The model under review builds one solid part; all positions refer to its coordinate system, in mm. A direction names the side the tool comes from. Coordinates: 2 decimals unless noted, no trailing zeros. Loops run counter-clockwise (first coordinate to the right, second up) from the corner with the lowest first, then second, coordinate; pieces in that order, holes last. Notation, with made-up numbers: (63, 44.25) - (105, 44.25) arc R15 cw to (105, 69.25) - close; hole circle Ø1 at (25, -18). An arc over 180 degrees is marked (long way). Use a Markdown table: item, result. Add a question column.
1) Add section C-C, the plane z = -13.5. Give the boundary of the cut face in (x, y).
2) The part is to be moulded in two halves that separate along X. For faces 4 (the flat face through (40, -4, 3)), 5 (the flat face through (2.6, 0.2, 85)), 6 (the cylindrical face through (-27.77, 2.03, 30.55)), say which applies: pulls with the +X half, pulls with the -X half, needs draft (parallel to the pull), parting line crosses it, or undercut.
3) Clearance check with flat-ended pins moving along their axes: pin 1 (6 mm diameter, centred on x = -8, y = -4, fed in from -Z); pin 2 (5 mm diameter, centred on x = 12, z = -38, fed in from -Y); pin 3 (3.5 mm diameter, centred on x = 9.5, y = -8, fed in from +Z). State where each tip first meets the part, or that it passes through.
4) Add section B-B, the plane y = -2.75. Give the boundary of the cut face in (x, z), and give its area (3 significant figures).
5) To check wall thickness, follow L1, parallel to X at y = 2.1, z = 45; L2, parallel to Z at x = -35.75, y = 2.75; L3, parallel to Z at x = 0, y = 2.25. State the ranges of each line that lie inside material, in increasing order. Write a range as [from, to].
6) Add section A-A, the plane x = 0. Give the boundary of the cut face in (y, z), and give its area (3 significant figures).
7) For faces 1 (the flat face through (35, -6, 66)), 2 (the flat face through (-1, -4, -85)), 3 (the cylindrical face through (37.556, -4.112, 44.599)), list the 3-axis set-ups (+Z, -Z, +X, -X, +Y, -Y) from which the entire face can be reached by the end or side of a thin tool; tool diameter is ignored.
8) Add section D-D, the plane z = 61. Give the boundary of the cut face in (x, y), and give its area (3 significant figures).
Autodesk Inventor part; units mm, degrees
ref_plane "YZ Plane" through (0, 0, 0) normal (1, 0, 0) x (0, 1, 0)
ref_plane "XZ Plane" through (0, 0, 0) normal (0, 1, 0) x (-1, 0, 0)
ref_plane "XY Plane" through (0, 0, 0) normal (0, 0, 1) x (1, 0, 0)
sketch "Sketch1" plane through (0, 0, 0) normal (0, 1, 0) x (-1, 0, 0)
  line L0 (40, 85) -> (-40, 85)
  line L1 (-40, 85) -> (-40, -85)
  line L2 (-40, -85) -> (40, -85)
  line L3 (40, -85) -> (40, 85)
  line L4 (40, 85) -> (-40, -85) construction
  line L5 (-40, 85) -> (40, -85) construction
  circle A0 centre (-40, -85) radius 6
  point P0 (0, 0)
  point P1 (-40, -79)
  point P2 (-34, -85)
  dimension "d0" = 80
  dimension "d1" = 170
  dimension "d2" = 12
extrude "Extrusion1" add sketch "Sketch1" along normal blind 4
sketch "Sketch2" plane through (0, 0, 0) normal (0, -1, 0) x (1, 0, 0)
  line L0 (40, 85) -> (40, -79)
  line L1 (-40, 85) -> (40, 85)
  line L2 (-40, -85) -> (-40, 85)
  line L3 (34, -85) -> (-40, -85)
  arc A0 (34, -85) -> (40, -79) centre (40, -85) ccw
  line L4 (35, 85) -> (35, -80)
  line L5 (35, -80) -> (-40, -80)
  point P0 (0, 0)
  dimension "d5" = 5
  dimension "d6" = 5
extrude "Extrusion2" add sketch "Sketch2" along normal blind 12 contours L0 A0 L3 L2 L5 L4 L1
sketch "Sketch3" plane through (0, 4, 0) normal (0, 1, 0) x (1, 0, 0)
  arc A0 (40, 79) -> (34, 85) centre (40, 85) ccw
  arc A1 (40, 79) -> (34, 85) centre (40, 85) ccw
  point P0 (0, 0)
hole "Hole1" at (40, 4, -85) direction (0, -1, 0) diameter 3.2 end through all
sketch "Sketch4" plane through (0, 4, 0) normal (0, 1, 0) x (1, 0, 0)
  line L0 (35.75, -45) -> (-35.75, -45) construction
  line L1 (-35.75, -45) -> (-35.75, 26.5) construction
  line L2 (-35.75, 26.5) -> (35.75, 26.5) construction
  line L3 (35.75, 26.5) -> (35.75, -45) construction
  line L4 (35.75, -45) -> (-35.75, 26.5) construction
  line L5 (-35.75, -45) -> (35.75, 26.5) construction
  circle A0 centre (40, 85) radius 1.6
  line L6 (40, -85) -> (40, 79)
  arc A1 (40, 79) -> (34, 85) centre (40, 85) ccw
  line L7 (34, 85) -> (-40, 85)
  line L8 (-40, 85) -> (-40, -85)
  line L9 (-40, -85) -> (40, -85)
  point P0 (0, 0)
  point P1 (0, -9.25)
  dimension "d16" = 71.5
  dimension "d17" = 40
hole "Hole2" at (-35.75, 4, 45) at (-35.75, 4, -26.5) at (35.75, 4, 45) at (35.75, 4, -26.5) direction (0, -1, 0) diameter 3.7 end through all
sketch "Sketch5" plane through (0, 4, 0) normal (0, 1, 0) x (1, 0, 0)
  circle A0 centre (0, -9.25) radius 35
  point P0 (0, 0)
  point P1 (0, -9.25)
  dimension "d25" = 70
extrude "Extrusion3" cut sketch "Sketch5" against normal up to surface (4 mm away)
fillet "Fillet1" radius 2 3 edges at (-40, -4, -85) (-40, 2, 85) (40, -4, 85)
equation "\"d6\" = d5"
properties part number "Power Box (12V) Cover" material "ABS Plastic"
From the geometry:
| question | item | result |
|---|---|---|
| 1 | outline | (-40, 0) - (-26.6, 0) - (-26.6, 4) - (-40, 4) - close; (26.6, 0) - (35, 0) - (35, -12) - (40, -12) - (40, 4) - (26.6, 4) - close |
| 2 | face 4 | pulls with the +X half |
| 2 | face 5 | needs draft |
| 2 | face 6 | undercut |
| 3 | pin 1 | stops at z = -85 |
| 3 | pin 2 | stops at y = 0 |
| 3 | pin 3 | stops at z = -80 |
| 4 | outline | (-40, -83) arc R2 ccw to (-38, -85) - (34, -85) arc R6 ccw (long way) to (40, -79) - (40, 83) arc R2 ccw to (38, 85) - (35, 85) - (35, 46.69) arc R1.85 cw (long way) to (35, 43.31) - (35, -24.81) arc R1.85 cw (long way) to (35, -28.19) - (35, -80) - (-40, -80) - close; hole circle Ø3.2 at (40, -85) |
| 4 | area | 1,280 mm^2 |
| 5 | L1 | x = [-40, -37.6], [-33.9, 33.9], [37.6, 40] |
| 5 | L2 | z = [-85, -28.35], [-24.65, 43.15], [46.85, 85] |
| 5 | L3 | z = [-85, -25.75], [44.25, 85] |
| 6 | outline | (-12, -85) - (4, -85) - (4, -25.75) - (0, -25.75) - (0, -80) - (-12, -80) - close; (0, 44.25) - (4, 44.25) - (4, 85) - (0, 85) - close |
| 6 | area | 460 mm^2 |
| 7 | face 1 | +Z, -X, -Y |
| 7 | face 2 | -Z, -X, +Y, -Y |
| 7 | face 3 | +Y, -Y |
| 8 | outline | (-40, 0) - (35, 0) - (35, -12) - (40, -12) - (40, 4) - (-40, 4) - close |
| 8 | area | 380 mm^2 |
